Check sheet for the modelled part. Datum: model origin and axes. Units: mm. Face numbers are marked on the shaded views. A direction names the side the tool comes from. Round coordinates to 2 decimals unless told otherwise and drop trailing zeros. Order: outer loops, then holes, each group sorted by start corner. A loop starts at its lowest first (then second) coordinate and runs counter-clockwise, first axis right, second up. Notation, with made-up numbers: M 87,28.25 L 145,28.25 A26 cw 145,65.25 Z; hole C 51,41.5 d2. An arc over 180 degrees is marked long. One line per item, written item: value. Start each with the question number.
(1) Cross-section at B-B, the plane y = -12. Enter the section's corners in (x, z), and give its area (3 significant figures).
(2) Release check for a two-part mould opening along Z. For the marked faces 1, 2, 3 and 4 record: released by +Z, released by -Z, zero draft, split by the parting line, or undercut.
(3) Depth check by flat-ended pin: pin 1 Ø1 at (x, z) = (36, 40) entering from +Y; pin 2 Ø7.5 at (x, z) = (30, 30) entering from -Y. Enter the tip coordinate at first touch or a pass-through.
(4) Cross-section at A-A, the plane x = 30. Enter the section's corners in (y, z) (3 decimals).
(5) Cross-section at D-D, the plane x = 44. Enter the section's corners in (y, z), and give its area (3 significant figures).
(6) Cross-section at C-C, the plane z = 30. Enter the section's corners in (x, y) (3 decimals).
(7) Thickness scan on L1, parallel to X at y = -8.5, z = 28.5; L2, parallel to Z at x = 30, y = -2.9 (3 decimals); L3, parallel to Y at x = 22, z = 41.5. Record the ranges inside material, lowest first.
(8) Access from +Z, -Z, +X, -X, +Y, -Y to the whole of each face (thin tool, end or side, straight path). Record for the marked faces 5 and 6.
from build123d import *

# Parameters (mm, degrees)
F0_W     = 60
F0_H     = 60
F0_W_2   = 40
F0_H_2   = 40
F1_DEPTH = 14
F0_R     = 3.175
F2_DEPTH = 4
F3_R     = 3


# Not quite as in the source:
# - a feature names something its author has since deleted; it is built from what else it names


with BuildPart() as f1:
    # F0 (on Front) → F1 (new body)
    with BuildSketch(Plane.XZ):
        with Locations((30, 30)):
            Rectangle(F0_W, F0_H)
        with Locations((30, 30)):
            Rectangle(F0_W_2, F0_H_2, mode=Mode.SUBTRACT)
    extrude(amount=F1_DEPTH)

    # F0 (on Front) → F2 (join)
    with BuildSketch(Plane.XZ):
        with Locations((30, 30)):
            Rectangle(F0_W_2, F0_H_2)
        with Locations((30, 30)):
            Circle(F0_R, mode=Mode.SUBTRACT)
    extrude(amount=F2_DEPTH)

    # F3
    f3_edges = [f1.edges().sort_by_distance(p)[0] for p in [
        (0, -7, 0),
        (0, -7, 60),
        (60, -7, 60),
        (60, -7, 0),
        (60, 0, 30),
        (30, 0, 60),
        (0, 0, 30),
        (30, 0, 0),
    ]]
    fillet(f3_edges, radius=F3_R)


solid = f1.part
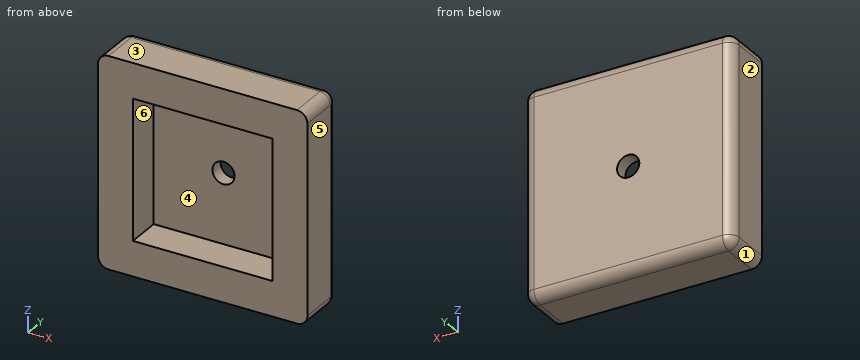
Values found:
1. outline: M 0,3 A3 ccw 3,0 L 57,0 A3 ccw 60,3 L 60,57 A3 ccw 57,60 L 3,60 A3 ccw 0,57 Z; hole M 10,10 L 50,10 L 50,50 L 10,50 Z
1. area: 1,990 mm^2
2. face 1: released by -Z
2. face 2: zero draft
2. face 3: released by +Z
2. face 4: undercut
3. pin 1: y = 0
3. pin 2: y = -4
4. outline: M -14,0 L -3,0 A3 ccw 0,3 L 0,26.825 L -4,26.825 L -4,10 L -14,10 Z; M -14,50 L -4,50 L -4,33.175 L 0,33.175 L 0,57 A3 ccw -3,60 L -14,60 Z
5. outline: M -14,0 L -3,0 A3 ccw 0,3 L 0,57 A3 ccw -3,60 L -14,60 L -14,50 L -4,50 L -4,10 L -14,10 Z
5. area: 436 mm^2
6. outline: M 0,-14 L 10,-14 L 10,-4 L 26.825,-4 L 26.825,0 L 3,0 A3 ccw 0,-3 Z; M 33.175,-4 L 50,-4 L 50,-14 L 60,-14 L 60,-3 A3 ccw 57,0 L 33.175,0 Z
7. L1: 0 to 10, 50 to 60
7. L2: 0.002 to 26.825, 33.175 to 59.998
7. L3: -4 to 0
8. face 5: +Z, -Z, +X, +Y, -Y
8. face 6: -Y
